Read the model definition and answer for the solid it produces. Units are mm, in the model's axes. A direction names the side the tool comes from. Coordinates: 2 decimals unless noted, no trailing zeros. Order: outer loops, then holes, each group sorted by start corner. A loop starts at its lowest first (then second) coordinate and runs counter-clockwise, first axis right, second up. Notation, with made-up numbers: (0.5, -30.5) -> (4.5, -30.5) arc R20 ccw to (4.5, -1.5) -> close; hole circle Ø4 at (-21, 39.5). An arc over 180 degrees is marked (long way). Answer in a Markdown table with one row per item.
from build123d import *

# Parameters (mm, degrees)
MODEL_R             = 5.191903136
MODEL_R_2           = 5.25
BOSS_EXTRUDE1_DEPTH = 5
BOSS_EXTRUDE2_DEPTH = 5
SKETCH3_R           = 51.25
CUT_EXTRUDE1_DEPTH  = 6


with BuildPart() as part:
    # Model → Boss-Extrude1 (new body)
    with BuildSketch(Plane.XY):
        with BuildLine():
            Line((869.6, 129.800004709), (854.6, 129.800004709))
            Line((854.6, 129.800004709), (854.6, 124.800004709))
            ThreePointArc((854.6, 124.800004709), (842.940279, 95.005240735), (815.123335737, 79.19718198))
            ThreePointArc((815.123335737, 79.19718198), (819.577050566, 70.004649675), (820.028101645, 59.800004709))
            Line((820.028101645, 59.800004709), (849.60000149, 59.800004709))
            ThreePointArc((849.60000149, 59.800004709), (852.428428615, 58.628431833), (853.60000149, 55.800004709))
            Line((853.60000149, 55.800004709), (853.60000149, 44.400154403))
            Line((853.60000149, 44.400154403), (856.099999799, 43.300004388))
            Line((856.099999799, 43.300004388), (853.60000149, 38.829377357))
            Line((853.60000149, 38.829377357), (853.60000149, -2.199993903))
            Line((853.60000149, -2.199993903), (869.6, -2.199993903))
            Line((869.6, -2.199993903), (869.6, 129.800004709))
        make_face()
        with Locations((861.6, 9.391497171)):
            Circle(MODEL_R, mode=Mode.SUBTRACT)
        with Locations((861.6, 114.800004709)):
            Circle(MODEL_R_2, mode=Mode.SUBTRACT)
    extrude(amount=BOSS_EXTRUDE1_DEPTH)

    # Sketch4 → Boss-Extrude2 (add)
    with BuildSketch(Plane.XY):
        Polygon((854.6, 129.800004709), (799.700462268, 74.900466976), (857.081865671, 78.451748184), (855.676639351, 119.436170701), (858.647890459, 128.484980891), align=None)
    extrude(amount=BOSS_EXTRUDE2_DEPTH)

    # Sketch3 → Cut-Extrude1 (cut)
    with BuildSketch(Plane(origin=(0, 0, 0), x_dir=(-1, 0, 0), z_dir=(0, 0, -1))):
        with Locations((-794.6, 64.800004709)):
            Circle(SKETCH3_R)
    extrude(amount=-CUT_EXTRUDE1_DEPTH, mode=Mode.SUBTRACT)


solid = part.part
Q1. The part is cut by section D-D (x = 833.5). Write down the section's boundary in (y, z).
Outcome:
| item | result |
|---|---|
| outline | (98.17, 0) -> (108.7, 0) -> (108.7, 5) -> (98.17, 5) -> close |
Q2. The part is cut by section B-B (z = 1.8). Write down the section's boundary in (x, y), then the cut area to 3 significant figures.
Outcome:
| item | result |
|---|---|
| outline | (828.25, 103.45) arc R51.25 cw to (845.61, 59.8) -> (849.6, 59.8) arc R4 cw to (853.6, 55.8) -> (853.6, 44.4) -> (856.1, 43.3) -> (853.6, 38.83) -> (853.6, -2.2) -> (869.6, -2.2) -> (869.6, 129.8) -> (854.6, 129.8) -> close; hole circle Ø10.5 at (861.6, 114.8); hole circle Ø10.38 at (861.6, 9.39) |
| area | 2,810 mm² |
Q3. For faces 1 (the face through (848, 59.8, 2)), 2 (the face through (869.6, 63, 2)), 3 (the face through (854.83, 43.86, 2.46)), determine the directions among +Z, -Z, +X, -X, +Y, -Y from which every point of the face is accessible in a straight line to the end or side of a thin tool.
Outcome:
| item | result |
|---|---|
| face 1 | +Z, -Z, -X, -Y |
| face 2 | +Z, -Z, +X, +Y, -Y |
| face 3 | +Z, -Z, -X |
Q4. For a pull along Y with two mould halves and no side action, classify faces 4 (the face through (853.6, 19, 2)), 5 (the face through (861, -2.2, 2)), 6 (the face through (854.87, 41.1, 2.46)) as pulls with the +Y half, pulls with the -Y half, needs draft (parallel to the pull), parting line crosses it, or undercut.
Outcome:
| item | result |
|---|---|
| face 4 | needs draft |
| face 5 | pulls with the -Y half |
| face 6 | undercut |
Q5. The part is cut by section A-A (x = 861.6). Write down the section's boundary in (y, z), then the cut area to 3 significant figures.
Outcome:
| item | result |
|---|---|
| outline | (-2.2, 0) -> (4.2, 0) -> (4.2, 5) -> (-2.2, 5) -> close; (14.58, 0) -> (109.55, 0) -> (109.55, 5) -> (14.58, 5) -> close; (120.05, 0) -> (129.8, 0) -> (129.8, 5) -> (120.05, 5) -> close |
| area | 556 mm² |
Q6. Given pin 1 (1 mm diameter, centred on y = 57.5, z = 2.5, fed in from -X); pin 2 (2 mm diameter, centred on x = 848.5, z = 1, fed in from +Y); pin 3 (8.5 mm diameter, centred on x = 861.6, y = 9.39, fed in from -Z), each flat-ended and moving along its own axis, determine where each tip first touches the part or whether it passes through.
Outcome:
| item | result |
|---|---|
| pin 1 | x = 852.94 |
| pin 2 | y = 124.7 |
| pin 3 | through |
Q7. The part is cut by section C-C (y = 10.5). Write down the section's boundary in (x, z).
Outcome:
| item | result |
|---|---|
| outline | (853.6, 0) -> (856.53, 0) -> (856.53, 5) -> (853.6, 5) -> close; (866.67, 0) -> (869.6, 0) -> (869.6, 5) -> (866.67, 5) -> close |
Q8. Consider line 1 (Y direction, x = 861.6, z = 3.05); line 2 (X direction, y = 38, z = 3.7); line 3 (X direction, y = 119, z = 0.45). Determine where each line is inside the solid, lowest interval first.
Outcome:
| item | result |
|---|---|
| line 1 | -2.2 to 4.2, 14.58 to 109.55, 120.05 to 129.8 |
| line 2 | 853.6 to 869.6 |
| line 3 | 843.8 to 858.45, 864.75 to 869.6 |
